Geometry check sheet. Reference: the model listing, model coordinates, mm. Round coordinates to 2 decimals unless told otherwise and drop trailing zeros. Order: outer loops, then holes, each group sorted by start corner. A loop starts at its lowest first (then second) coordinate and runs counter-clockwise, first axis right, second up.
(1) Sectioned sample at A-A (z = -100.5). Record the boundary of the cut face in (x, y) (3 decimals).
(2) Go/stop test with a flat-tipped pin: pin 1 (5 mm diameter, centred on x = 15, z = 217.425, fed in from -Y). Record where the tip stops, or that it passes through.
(3) Material ranges on line 1 along X through (y, z) = (0.55, -8); line 2 along Z through (x, y) = (-15, 1.7) (3 decimals); line 3 along X through (y, z) = (0.85, 196), recorded low to high.
(4) Sectioned sample at B-B (y = 2.15). Record the boundary of the cut face in (x, z) (3 decimals), plus the area to 3 significant figures.
from build123d import *

# Parameters (mm, degrees)
SKETCH1_W            = 50
SKETCH1_H            = 457.2
BOSS_EXTRUDE1_DEPTH  = 3.175
CUT_EXTRUDE1_DEPTH   = 230.984870426
M3_CLEARANCE_HOLE1_D = 3.2


with BuildPart() as part:
    # Sketch1 → Boss-Extrude1 (new body)
    with BuildSketch(Plane(origin=(0, 0, 0), x_dir=(1, 0, 0), z_dir=(0, 1, 0))):
        Rectangle(SKETCH1_W, SKETCH1_H)
    extrude(amount=BOSS_EXTRUDE1_DEPTH)

    # Sketch2 → Cut-Extrude1 (cut, through all)
    with BuildSketch(Plane.XZ):
        with BuildLine():
            Line((-10.9, -3.6), (-10.9, -203.6))
            ThreePointArc((-10.9, -203.6), (-12.5, -205.2), (-14.1, -203.6))
            Line((-14.1, -203.6), (-14.1, -3.6))
            ThreePointArc((-14.1, -3.6), (-12.5, -2), (-10.9, -3.6))
        make_face()
        with BuildLine():
            Line((10.9, -3.6), (10.9, -203.6))
            ThreePointArc((10.9, -203.6), (12.5, -205.2), (14.1, -203.6))
            Line((14.1, -203.6), (14.1, -3.6))
            ThreePointArc((14.1, -3.6), (12.5, -2), (10.9, -3.6))
        make_face()
    extrude(amount=-CUT_EXTRUDE1_DEPTH, mode=Mode.SUBTRACT)

    # M3 Clearance Hole1 (through all)
    with Locations(Plane(origin=(0, 0, 0), x_dir=(-1, 0, 0), z_dir=(0, -1, 0))):
        with Locations((15, -217.425), (-15, -197.425), (-15, -217.425), (15, -197.425)):
            Hole(M3_CLEARANCE_HOLE1_D / 2)


solid = part.part
Answer below:
1. outline: (-25, 0) - (-14.1, 0) - (-14.1, 3.175) - (-25, 3.175) - close; (-10.9, 0) - (10.9, 0) - (10.9, 3.175) - (-10.9, 3.175) - close; (14.1, 0) - (25, 0) - (25, 3.175) - (14.1, 3.175) - close
2. pin 1: stops at y = 0
3. line 1: x = -25 to -14.1, -10.9 to 10.9, 14.1 to 25
3. line 2: z = -228.6 to 195.825, 199.025 to 215.825, 219.025 to 228.6
3. line 3: x = -25 to -15.73, -14.27 to 14.27, 15.73 to 25
4. outline: (-25, -228.6) - (25, -228.6) - (25, 228.6) - (-25, 228.6) - close; hole circle Ø3.2 at (-15, 197.425); hole circle Ø3.2 at (-15, 217.425); hole (-14.1, -203.6) arc R1.6 ccw to (-10.9, -203.6) - (-10.9, -3.6) arc R1.6 ccw to (-14.1, -3.6) - close; hole (10.9, -203.6) arc R1.6 ccw to (14.1, -203.6) - (14.1, -3.6) arc R1.6 ccw to (10.9, -3.6) - close; hole circle Ø3.2 at (15, 197.425); hole circle Ø3.2 at (15, 217.425)
4. area: 21,500 mm2
